from build123d import *

# Parameters (mm, degrees)
SKETCH1_R           = 2.413
BOSS_EXTRUDE1_DEPTH = 3.175
SKETCH2_W           = 22.86
SKETCH2_H           = 3.175
BOSS_EXTRUDE2_DEPTH = 25.4
CHAMFER1_SIZE       = 2.54


with BuildPart() as part:
    # Sketch1 → Boss-Extrude1 (new body)
    with BuildSketch(Plane(origin=(0, 0, 0), x_dir=(1, 0, 0), z_dir=(0, 1, 0))):
        Polygon((-27.94, -11.43), (27.94, -11.43), (27.94, 11.43), (11.43, 11.43), (11.43, 110.49), (-11.43, 110.49), (-11.43, 11.43), (-27.94, 11.43), align=None)
        with Locations((-22.7965, 0)):
            Circle(SKETCH1_R, mode=Mode.SUBTRACT)
        with Locations((22.7965, 0)):
            Circle(SKETCH1_R, mode=Mode.SUBTRACT)
    extrude(amount=BOSS_EXTRUDE1_DEPTH)

    # Sketch2 → Boss-Extrude2 (add)
    with BuildSketch(Plane(origin=(0, 3.175, 0), x_dir=(1, 0, 0), z_dir=(0, 1, 0))):
        with Locations((0, 108.9025)):
            Rectangle(SKETCH2_W, SKETCH2_H)
    extrude(amount=BOSS_EXTRUDE2_DEPTH)

    # Chamfer1
    chamfer1_edges = [part.edges().sort_by_distance(p)[0] for p in [
        (0, 28.575, -107.315),
    ]]
    chamfer(chamfer1_edges, length=CHAMFER1_SIZE)


solid = part.part
Design review of the part built by this model. Coordinates are the model's own, in mm. A direction names the side the tool comes from. Coordinates: 2 decimals unless noted, no trailing zeros. Loops run counter-clockwise (first coordinate to the right, second up) from the corner with the lowest first, then second, coordinate; pieces in that order, holes last. Notation, with made-up numbers: (39.5, 22.25) -> (63.5, 22.25) arc R26 cw to (63.5, 38.25) -> close; hole circle Ø11 at (13.5, 78). An arc over 180 degrees is marked (long way). Use a Markdown table: item, result. Add a question column.
Item 1: Wall thickness on L1, parallel to X at y = 0.65, z = 0; L2, parallel to Y at x = 14.5, z = -5 (3 decimals); L3, parallel to Z at x = 1.5, y = 20.5 (3 decimals): over which ranges is each line inside the solid? List them lowest first. Write a range as from..to.
Item 2: We need section D-D, the plane z = -102. Write out the cut boundary in (x, y) (3 decimals).
Item 3: We need section C-C, the plane y = 9. Write out the cut boundary in (x, z) (3 decimals).
Item 4: The part is to be moulded in two halves that separate along Z. For faces 1 (the flat face through (0, 14, -107.315)), 2 (the cylindrical face through (-25.207, 1.565, -0.106)), 3 (the cylindrical face through (20.386, 1.565, -0.106)), 4 (the flat face through (0, 14, -110.49)), say which applies: +Z half, -Z half, draft (parallel to the pull), parting line (faces both ways), or undercut.
Item 5: We need section B-B, the plane x = 7. Write out the cut boundary in (y, z) (3 decimals), and give its area (3 significant figures).
Item 6: Machinability: for faces 5 (the flat face through (-11.43, 3, -72)), 6 (the flat face through (0, 3.175, -36)), 7 (the flat face through (11.43, 3, -72)), which of the approach directions +Z, -Z, +X, -X, +Y, -Y give a long, thin tool a straight path to every point of the face, cutting with its end or side? Answer none if there is none.
Item 7: Clearance check with flat-ended pins moving along their axes: P1, Ø8, axis at x = 2, y = 12.5, coming from the +Z side (3 decimals); P2, Ø6.5, axis at x = -22.8, z = 0, coming from the +Y side (3 decimals); P3, Ø1, axis at x = 16.5, y = 2.5, coming from the -Z side. State where each tip first meets the part, or that it passes through.
Item 8: We need section A-A, the plane z = 0. Write out the cut boundary in (x, y) (1 decimal), and give its area (3 significant figures).
Numbers:
| question | item | result |
|---|---|---|
| 1 | L1 | x = -27.94..-25.21, -20.38..20.38, 25.21..27.94 |
| 1 | L2 | y = 0..3.175 |
| 1 | L3 | z = -110.49..-107.315 |
| 2 | outline | (-11.43, 0) -> (11.43, 0) -> (11.43, 3.175) -> (-11.43, 3.175) -> close |
| 3 | outline | (-11.43, -110.49) -> (11.43, -110.49) -> (11.43, -107.315) -> (-11.43, -107.315) -> close |
| 4 | face 1 | +Z half |
| 4 | face 2 | undercut |
| 4 | face 3 | undercut |
| 4 | face 4 | -Z half |
| 5 | outline | (0, -110.49) -> (28.575, -110.49) -> (28.575, -109.855) -> (26.035, -107.315) -> (3.175, -107.315) -> (3.175, 11.43) -> (0, 11.43) -> close |
| 5 | area | 465 mm^2 |
| 6 | face 5 | -Z, -X, +Y, -Y |
| 6 | face 6 | +Z, +X, -X, +Y |
| 6 | face 7 | -Z, +X, +Y, -Y |
| 7 | P1 | stops at z = -107.315 |
| 7 | P2 | stops at y = 3.175 |
| 7 | P3 | stops at z = -11.43 |
| 8 | outline | (-27.9, 0) -> (-25.2, 0) -> (-25.2, 3.2) -> (-27.9, 3.2) -> close; (-20.4, 0) -> (20.4, 0) -> (20.4, 3.2) -> (-20.4, 3.2) -> close; (25.2, 0) -> (27.9, 0) -> (27.9, 3.2) -> (25.2, 3.2) -> close |
| 8 | area | 147 mm^2 |
